Read the model definition and answer for the solid it produces. Units are mm, in the model's axes. Face numbers are marked on the shaded views. A direction names the side the tool comes from. Coordinates: 2 decimals unless noted, no trailing zeros. Write each loop counter-clockwise with the first axis right and the second up, starting at its lowest first coordinate (ties: lowest second). Pieces come first, ordered by that corner, then holes.
Item 1: Section C-C (x = -27) is taken. Give the vertices of the cut face in (y, z).
Item 2: A tool of negligible diameter and unlimited length cuts with its end or side. For the marked faces 1 and 2, from which of +Z, -Z, +X, -X, +Y, -Y can it reach the whole face along a straight path? Write none if from no direction.
Item 3: Section B-B (y = 53) is taken. Give the vertices of the cut face in (x, z), then the cut area to 3 significant figures.
Item 4: Straight lines are drawn through the part: probe 1 along Y at (x, z) = (-16.5, 4.5); probe 2 along Y at (x, z) = (32.5, 4.5); probe 3 along Y at (x, z) = (-32.5, 2.25). For each, find the intervals that lie inside material, in ascending order.
Item 5: Each of these flat-tipped pins is pushed along its axis until it touches: P1, Ø3, axis at x = -32.5, y = 10.17, coming from the -Z side; P2, Ø5, axis at x = 32.5, y = 11, coming from the +Z side; P3, Ø5, axis at x = 7.5, z = 8, coming from the +Y side. Where does it stop, or does it pass through?
Item 6: Section A-A (x = -16.5) is taken. Give the vertices of the cut face in (y, z).
Item 7: Section D-D (x = 18) is taken. Give the vertices of the cut face in (y, z).
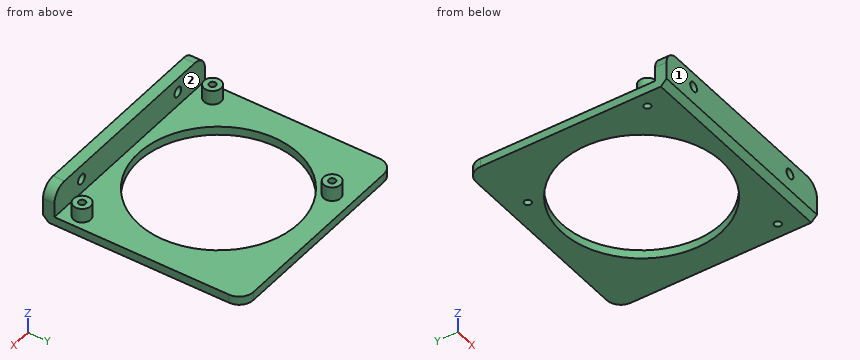
from build123d import *

# Parameters (mm, degrees)
SKETCH_W        = 75
SKETCH_H        = 70
PAD_DEPTH       = 3
SKETCH001_W     = 75
SKETCH001_H     = 4
PAD001_DEPTH    = 10
SKETCH002_R     = 3
PAD002_DEPTH    = 5
SKETCH003_R     = 1.2
POCKET_DEPTH    = 8.001
SKETCH004_R     = 1.7
POCKET001_DEPTH = 5
SKETCH005_R     = 27.911549
POCKET002_DEPTH = 5
FILLET_R        = 5
CHAMFER_SIZE    = 2


with BuildPart() as part:
    # Sketch → Pad (new body)
    with BuildSketch(Plane.XY):
        with Locations((0, 35)):
            Rectangle(SKETCH_W, SKETCH_H)
    extrude(amount=PAD_DEPTH)

    # Sketch001 → Pad001 (new body)
    with BuildSketch(Plane.XY.offset(3)):
        with Locations((0, 2)):
            Rectangle(SKETCH001_W, SKETCH001_H)
    extrude(amount=PAD001_DEPTH)

    # Sketch002 → Pad002 (new body)
    with BuildSketch(Plane.XY.offset(3)):
        with Locations((-16.5, 63.173148)):
            Circle(SKETCH002_R)
        with Locations((32.5, 10.173148)):
            Circle(SKETCH002_R)
        with Locations((-32.5, 10.173148)):
            Circle(SKETCH002_R)
    extrude(amount=PAD002_DEPTH)

    # Sketch003 → Pocket (cut, through all)
    with BuildSketch(Plane.XY.offset(8)):
        with Locations((-16.5, 63.173148)):
            Circle(SKETCH003_R)
        with Locations((32.5, 10.173148)):
            Circle(SKETCH003_R)
        with Locations((-32.5, 10.173148)):
            Circle(SKETCH003_R)
    extrude(amount=-POCKET_DEPTH, mode=Mode.SUBTRACT)

    # Sketch004 → Pocket001 (cut)
    with BuildSketch(Plane(origin=(0, 4, 0), x_dir=(-1, 0, 0), z_dir=(0, 1, 0))):
        with Locations((-24, 8)):
            Circle(SKETCH004_R)
        with Locations((24, 8)):
            Circle(SKETCH004_R)
    extrude(amount=-POCKET001_DEPTH, mode=Mode.SUBTRACT)

    # Sketch005 → Pocket002 (cut)
    with BuildSketch(Plane.XY.offset(3)):
        with Locations((0, 34.999702)):
            Circle(SKETCH005_R)
    extrude(amount=-POCKET002_DEPTH, mode=Mode.SUBTRACT)

    # Fillet
    fillet_edges = [part.edges().sort_by_distance(p)[0] for p in [
        (-37.5, 70, 1.5),
        (37.5, 70, 1.5),
        (37.5, 2, 13),
        (-37.5, 2, 13),
    ]]
    fillet(fillet_edges, radius=FILLET_R)

    # Chamfer
    chamfer_edges = [part.edges().sort_by_distance(p)[0] for p in [
        (0, 0, 0),
    ]]
    chamfer(chamfer_edges, length=CHAMFER_SIZE)


solid = part.part
Established:
1. outline: (0, 2) - (2, 0) - (27.92, 0) - (27.92, 3) - (4, 3) - (4, 13) - (0, 13) - close; (42.07, 0) - (70, 0) - (70, 3) - (42.07, 3) - close
2. face 1: +Z, -Z, +X, -X, -Y
2. face 2: +Z, +X, -X
3. outline: (-37.5, 0) - (-21.33, 0) - (-21.33, 3) - (-37.5, 3) - close; (21.33, 0) - (37.5, 0) - (37.5, 3) - (21.33, 3) - close
3. area: 97.0 mm2
4. probe 1: y = 0 to 4, 60.17 to 61.97, 64.37 to 66.17
4. probe 2: y = 0 to 4, 7.17 to 8.97, 11.37 to 13.17
4. probe 3: y = 0 to 8.97, 11.37 to 70
5. P1: stops at z = 0
5. P2: stops at z = 8
5. P3: stops at y = 4
6. outline: (0, 2) - (2, 0) - (12.49, 0) - (12.49, 3) - (4, 3) - (4, 13) - (0, 13) - close; (57.51, 0) - (61.97, 0) - (61.97, 8) - (60.17, 8) - (60.17, 3) - (57.51, 3) - close; (64.37, 0) - (70, 0) - (70, 3) - (66.17, 3) - (66.17, 8) - (64.37, 8) - close
7. outline: (0, 2) - (2, 0) - (13.67, 0) - (13.67, 3) - (4, 3) - (4, 13) - (0, 13) - close; (56.33, 0) - (70, 0) - (70, 3) - (56.33, 3) - close
